The model under review builds one solid part; all positions refer to its coordinate system, in mm. Face numbers are marked on the shaded views. A direction names the side the tool comes from. Round coordinates to 2 decimals unless told otherwise and drop trailing zeros. Order: outer loops, then holes, each group sorted by start corner. A loop starts at its lowest first (then second) coordinate and runs counter-clockwise, first axis right, second up.
1) Clearance check with flat-ended pins moving along their axes: P1, Ø16, axis at x = 148.5, y = 11, coming from the +Z side; P2, Ø10, axis at y = 11.5, z = 155, coming from the -X side; P3, Ø10, axis at x = 165, z = 158.5, coming from the -Y side. State where each tip first meets the part, or that it passes through.
2) Consider section A-A (x = 38.5). Give the boundary of the cut face in (y, z), then the cut area to 3 significant figures.
3) To check wall thickness, follow L1, parallel to Z at x = 39.5, y = 7. State the ranges of the line that lie inside material, in increasing order.
4) Machinability: for the marked faces 1, 2 and 3, which of the approach directions +Z, -Z, +X, -X, +Y, -Y give a long, thin tool a straight path to every point of the face, cutting with its end or side? Answer none if there is none.
Autodesk Fusion 360 part; units mm, degrees
sketch "Sketch1" plane through (0, 0, 0) normal (0, 0, 1) x (1, 0, 0)
  line L0 (0, 0) -> (183, 0)
  line L1 (183, 0) -> (183, 77)
  line L2 (183, 77) -> (0, 77)
  line L3 (0, 77) -> (0, 0)
  dimension "d1" = 183
  dimension "d2" = 77
extrude "Extrude1" add sketch "Sketch1" along normal blind 169
sketch "Sketch2" plane through (0, 0, 169) normal (0, 0, 1) x (-1, 0, 0)
  line L0 (0, -77) -> (0, 0)
  line L1 (0, 0) -> (-183, 0)
  line L2 (-183, 0) -> (-183, -77)
  line L3 (-183, -77) -> (0, -77)
  line L4 (0, -20) -> (-60, -20)
  line L5 (-60, -20) -> (-60, 0)
  line L6 (-60, 0) -> (0, 0)
  line L7 (0, 0) -> (0, -20)
  line L8 (-183, 0) -> (-123, 0)
  line L9 (-123, 0) -> (-123, -20)
  line L10 (-123, -20) -> (-183, -20)
  line L11 (-183, -20) -> (-183, 0)
  dimension "d5" = 60
extrude "Extrude2" cut sketch "Sketch2" against normal blind 20 contours L0 L1 L4 L5 L6 L7 | L1 L2 L8 L9 L10 L11
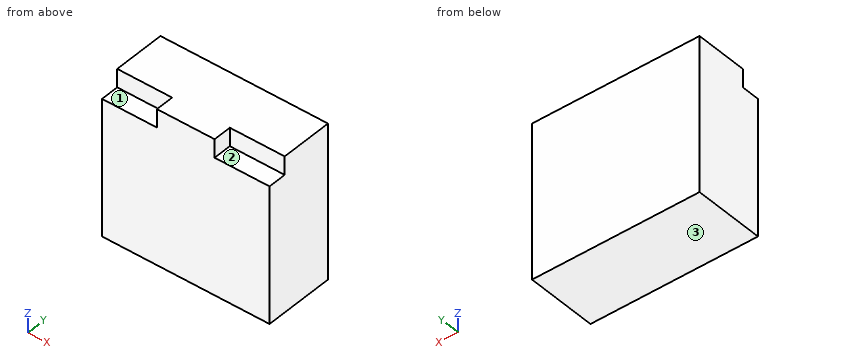
Answer below:
1. P1: stops at z = 149
1. P2: stops at x = 60
1. P3: stops at y = 20
2. outline: (0, 0) - (77, 0) - (77, 169) - (20, 169) - (20, 149) - (0, 149) - close
2. area: 12,600 mm2
3. L1: z = 0 to 149
4. face 1: +Z, -X, -Y
4. face 2: +Z, +X, -Y
4. face 3: -Z, +X, -X, +Y, -Y
